Source: CAD feature listing. Evaluate the final solid. Frame: model axes, mm. A direction names the side the tool comes from. Coordinates: 2 decimals unless noted, no trailing zeros. Order: outer loops, then holes, each group sorted by start corner. A loop starts at its lowest first (then second) coordinate and runs counter-clockwise, first axis right, second up.
Item 1: Section A-A on z = 17.5. Return the cut outline in (x, y), then the cut area to 3 significant figures.
Item 2: Ray query, line 1 (X direction, y = 5.75, z = -17.5); line 2 (Z direction, x = -11.5, y = 5.25); line 3 (Y direction, x = 15.5, z = 28.5). Return the intervals inside material, ascending.
Item 3: Contact query for flat-ended pins moving along their axis: P1, Ø1.5, axis at x = -7.5, y = 7.5, coming from the +Z side; P2, Ø1.5, axis at y = 3, z = 33, coming from the +X side; P3, Ø1.9, axis at x = -12, z = 17.5, coming from the -Y side; P4, Ø4, axis at x = 12, z = -17.5, coming from the +Y side. Output: stop coordinate, or through.
Item 4: Section B-B on x = -12. Return the cut outline in (y, z).
Item 5: Mould query, pull axis Z, two halves, no side actions, for faces 4 (the flat face through (0, 2, 40)), 5 (the cylindrical face through (-12.97, 5.07, -18.77)), 6 (the flat face through (0, 10, 0)). Classes: released by +Z, released by -Z, zero draft, split by the parting line, or undercut.
Item 6: Section C-C on y = 3.5. Return the cut outline in (x, z).
Item 7: Section D-D on z = -17. Return the cut outline in (x, y), then the cut area to 3 significant figures.
Item 8: Reachability of faces 1 (the cylindrical face through (-17.4, 4.93, -24.43)), 2 (the flat face through (0, 7, 25)), 3 (the flat face through (17, 2, 31)) from +Z, -Z, +X, -X, +Y, -Y: full face, straight path, thin tool, end or side. Return the list, or none.
from build123d import *

# Parameters (mm, degrees)
SKETCH_1_W          = 36
SKETCH_1_H          = 50
SKETCH_1_W_2        = 34
SKETCH_1_H_2        = 15
EXTRUDE_1_DEPTH     = 10
SKETCH_2_R          = 1.6
CUT_EXTRUDE_1_DEPTH = 10
SKETCH_3_W          = 34
SKETCH_3_H          = 15
CUT_EXTRUDE_2_DEPTH = 5
FILLET_1_R          = 2


with BuildPart() as part:
    # 草图1 → 凸台-拉伸1 (new body)
    with BuildSketch(Plane(origin=(0, 0, 0), x_dir=(1, 0, 0), z_dir=(0, 1, 0))):
        Rectangle(SKETCH_1_W, SKETCH_1_H)
        with Locations((0, -32.5)):
            Rectangle(SKETCH_1_W_2, SKETCH_1_H_2)
    extrude(amount=EXTRUDE_1_DEPTH)

    # 草图2 → 切除-拉伸1 (cut)
    with BuildSketch(Plane(origin=(0, 10, 0), x_dir=(1, 0, 0), z_dir=(0, 1, 0))):
        with Locations(Location((12, 17.5, 0), (0, 0, 270))):
            Circle(SKETCH_2_R)
        with Locations(Location((-12, 17.5, 0), (0, 0, 270))):
            Circle(SKETCH_2_R)
        with Locations(Location((-12, -17.5, 0), (0, 0, 270))):
            Circle(SKETCH_2_R)
        with Locations(Location((12, -17.5, 0), (0, 0, 270))):
            Circle(SKETCH_2_R)
    extrude(amount=-CUT_EXTRUDE_1_DEPTH, mode=Mode.SUBTRACT)

    # 草图3 → 切除-拉伸2 (cut)
    with BuildSketch(Plane(origin=(0, 10, 0), x_dir=(1, 0, 0), z_dir=(0, 1, 0))):
        with Locations((0, -32.5)):
            Rectangle(SKETCH_3_W, SKETCH_3_H)
    extrude(amount=-CUT_EXTRUDE_2_DEPTH, mode=Mode.SUBTRACT)

    # 圆角1
    # the kernel refuses this fillet: 2 mm, written as the material it takes off along each edge
    with BuildSketch(Plane(origin=(18, -5, -25), x_dir=(0, 0, 1), z_dir=(0, 1, 0))) as fillet_1_piece_1:
        with BuildLine():
            CenterArc((FILLET_1_R, -FILLET_1_R), FILLET_1_R, 90, 90)
            Line((0, -FILLET_1_R), (0, 0))
            Line((0, 0), (FILLET_1_R, 0))
        make_face()
    extrude(amount=20, mode=Mode.SUBTRACT)
    with BuildSketch(Plane(origin=(17, -5, 40), x_dir=(-1, 0, 0), z_dir=(0, 1, 0)), Plane(origin=(-17, -5, 40), x_dir=(0, 0, -1), z_dir=(0, 1, 0))) as fillet_1_piece_2:
        with BuildLine():
            CenterArc((FILLET_1_R, -FILLET_1_R), FILLET_1_R, 90, 90)
            Line((0, -FILLET_1_R), (0, 0))
            Line((0, 0), (FILLET_1_R, 0))
        make_face()
    extrude(amount=15, mode=Mode.SUBTRACT)
    with BuildSketch(Plane(origin=(-18, -5, 25), x_dir=(0, 0, -1), z_dir=(0, 1, 0))) as fillet_1_piece_3_section:
        with BuildLine():
            CenterArc((FILLET_1_R, -FILLET_1_R), FILLET_1_R, 90, 90)
            Line((0, -FILLET_1_R), (0, 0))
            Line((0, 0), (FILLET_1_R, 0))
        make_face()
    fillet_1_piece_3 = extrude(amount=20, mode=Mode.PRIVATE)
    fillet_1_piece_3 = split(fillet_1_piece_3, bisect_by=Plane(origin=(-17, 2.5, 24.511950301), z_dir=(-1, 0, 0)), keep=Keep.TOP, mode=Mode.PRIVATE)
    add(fillet_1_piece_3, mode=Mode.SUBTRACT)
    with BuildSketch(Plane(origin=(-18, -5, 25), x_dir=(0, 0, -1), z_dir=(0, 1, 0))) as fillet_1_piece_4_section:
        with BuildLine():
            CenterArc((FILLET_1_R, -FILLET_1_R), FILLET_1_R, 90, 90)
            Line((0, -FILLET_1_R), (0, 0))
            Line((0, 0), (FILLET_1_R, 0))
        make_face()
    fillet_1_piece_4 = extrude(amount=20, mode=Mode.PRIVATE)
    fillet_1_piece_4 = split(fillet_1_piece_4, bisect_by=Plane(origin=(-16.753472775, 5, 24.920630815), z_dir=(0, 1, 0)), keep=Keep.TOP, mode=Mode.PRIVATE)
    add(fillet_1_piece_4, mode=Mode.SUBTRACT)
    with BuildSketch(Plane(origin=(18, -5, 25), x_dir=(0, 0, -1), z_dir=(0, 1, 0))) as fillet_1_piece_5_section:
        with BuildLine():
            CenterArc((FILLET_1_R, FILLET_1_R), FILLET_1_R, 180, 90)
            Line((0, FILLET_1_R), (0, 0))
            Line((0, 0), (FILLET_1_R, 0))
        make_face()
    fillet_1_piece_5 = extrude(amount=20, mode=Mode.PRIVATE)
    fillet_1_piece_5 = split(fillet_1_piece_5, bisect_by=Plane(origin=(17, 2.5, 24.511950301), z_dir=(1, 0, 0)), keep=Keep.TOP, mode=Mode.PRIVATE)
    add(fillet_1_piece_5, mode=Mode.SUBTRACT)
    with BuildSketch(Plane(origin=(18, -5, 25), x_dir=(0, 0, -1), z_dir=(0, 1, 0))) as fillet_1_piece_6_section:
        with BuildLine():
            CenterArc((FILLET_1_R, FILLET_1_R), FILLET_1_R, 180, 90)
            Line((0, FILLET_1_R), (0, 0))
            Line((0, 0), (FILLET_1_R, 0))
        make_face()
    fillet_1_piece_6 = extrude(amount=20, mode=Mode.PRIVATE)
    fillet_1_piece_6 = split(fillet_1_piece_6, bisect_by=Plane(origin=(16.753472775, 5, 24.920630815), z_dir=(0, 1, 0)), keep=Keep.TOP, mode=Mode.PRIVATE)
    add(fillet_1_piece_6, mode=Mode.SUBTRACT)
    with BuildSketch(Plane(origin=(-18, -5, -25), x_dir=(0, 0, 1), z_dir=(0, 1, 0))) as fillet_1_piece_7:
        with BuildLine():
            CenterArc((FILLET_1_R, FILLET_1_R), FILLET_1_R, 180, 90)
            Line((0, FILLET_1_R), (0, 0))
            Line((0, 0), (FILLET_1_R, 0))
        make_face()
    extrude(amount=20, mode=Mode.SUBTRACT)


solid = part.part
Answer list:
1. outline: (-18, 0) - (-13.6, 0) - (-13.6, 10) - (-18, 10) - close; (-10.4, 0) - (10.4, 0) - (10.4, 10) - (-10.4, 10) - close; (13.6, 0) - (18, 0) - (18, 10) - (13.6, 10) - close
1. area: 296 mm2
2. line 1: x = -18 to -13.6, -10.4 to 10.4, 13.6 to 18
2. line 2: z = -25 to -19.02, -15.98 to 15.98, 19.02 to 25
2. line 3: y = 0 to 5
3. P1: stops at z = 25
3. P2: stops at x = 17
3. P3: passes through
3. P4: stops at y = 10
4. outline: (0, -25) - (10, -25) - (10, -19.1) - (0, -19.1) - close; (0, -15.9) - (10, -15.9) - (10, 15.9) - (0, 15.9) - close; (0, 19.1) - (10, 19.1) - (10, 25) - (5, 25) - (5, 40) - (0, 40) - close
5. face 4: released by +Z
5. face 5: undercut
5. face 6: zero draft
6. outline: (-18, -23) arc R2 ccw to (-16, -25) - (16, -25) arc R2 ccw to (18, -23) - (18, 23) arc R2 ccw to (17, 24.73) - (17, 38) arc R2 ccw to (15, 40) - (-15, 40) arc R2 ccw to (-17, 38) - (-17, 24.73) arc R2 ccw to (-18, 23) - close; hole circle Ø3.2 at (-12, -17.5); hole circle Ø3.2 at (-12, 17.5); hole circle Ø3.2 at (12, -17.5); hole circle Ø3.2 at (12, 17.5)
7. outline: (-18, 0) - (-13.52, 0) - (-13.52, 10) - (-18, 10) - close; (-10.48, 0) - (10.48, 0) - (10.48, 10) - (-10.48, 10) - close; (13.52, 0) - (18, 0) - (18, 10) - (13.52, 10) - close
7. area: 299 mm2
8. face 1: -Z, -X, +Y, -Y
8. face 2: +Z, +X, -X, +Y
8. face 3: +Z, +X, +Y, -Y
